```python
from build123d import *

# Parameters (mm, degrees)
SKETCH1_W           = 46.99
SKETCH1_H           = 12.7
SKETCH1_R           = 1.5875
SKETCH1_R_2         = 1.6129
BOSS_EXTRUDE1_DEPTH = 5.715
SKETCH2_R           = 2.921
CUT_EXTRUDE1_DEPTH  = 3.302
FILLET1_R           = 2.54
FILLET2_R           = 0.254


with BuildPart() as part:
    # Sketch1 → Boss-Extrude1 (new body)
    with BuildSketch(Plane(origin=(0, 0, 0), x_dir=(0, 0, -1), z_dir=(1, 0, 0))):
        Rectangle(SKETCH1_W, SKETCH1_H)
        with Locations((-19.05, 0)):
            Circle(SKETCH1_R, mode=Mode.SUBTRACT)
        with Locations(Location((19.05, 0, 0), (0, 0, 180))):
            Circle(SKETCH1_R, mode=Mode.SUBTRACT)
        with Locations((-4.028538113, -1.878538173)):
            Circle(SKETCH1_R_2, mode=Mode.SUBTRACT)
        with Locations((4.028538113, 1.878538173)):
            Circle(SKETCH1_R_2, mode=Mode.SUBTRACT)
    extrude(amount=BOSS_EXTRUDE1_DEPTH)

    # Sketch2 → Cut-Extrude1 (cut)
    with BuildSketch(Plane(origin=(5.715, 0, 0), x_dir=(0, 0, -1), z_dir=(1, 0, 0))):
        with Locations((-4.028538113, -1.878538173)):
            Circle(SKETCH2_R)
        with Locations((4.028538113, 1.878538173)):
            Circle(SKETCH2_R)
    extrude(amount=-CUT_EXTRUDE1_DEPTH, mode=Mode.SUBTRACT)

    # Fillet1
    fillet1_edges = [part.edges().sort_by_distance(p)[0] for p in [
        (2.8575, 6.35, 23.495),
        (2.8575, 6.35, -23.495),
        (2.8575, -6.35, -23.495),
        (2.8575, -6.35, 23.495),
    ]]
    fillet(fillet1_edges, radius=FILLET1_R)

    # Fillet2
    fillet2_edges = [part.edges().sort_by_distance(p)[0] for p in [
        (2.413, -1.878538173, 6.949538113),
        (2.413, 1.878538173, -1.107538113),
    ]]
    fillet(fillet2_edges, radius=FILLET2_R)


solid = part.part
```
Verification items for the finished model (mm, model axes). A direction names the side the tool comes from. Coordinates: 2 decimals unless noted, no trailing zeros. Write item = value, one per line.
Q1. Go/stop test with a flat-tipped pin: pin 1 Ø3.5 at (y, z) = (1.88, -4.03) entering from +X. Record where the tip stops, or that it passes through.
Answer:
pin_1 = 2.41
Q2. Cross-section at B-B (x = 4.6). Give the number of separate pieces and of enclosed holes in the cut face, plus the area to 3 significant figures.
Answer:
separate_pieces = 1
enclosed_holes = 4
area = 522 mm²
Q3. Mould release check, pull along Y, two halves, no side actions. Record for faces 3 (the face through (3, 0, 23.495)), 4 (the face through (4.21, 4.34, -5.6)), 5 (the face through (1.19, 2.97, -2.84)), 6 (the face through (2.898, -5.626, -22.731)): released by +Y, released by -Y, zero draft, split by the parting line, or undercut.
Answer:
face_3 = zero draft
face_4 = undercut
face_5 = undercut
face_6 = released by -Y
Q4. Access from +Z, -Z, +X, -X, +Y, -Y to the whole of each face (thin tool, end or side, straight path). Record for faces 1 (the face through (2.898, 5.586, 22.771)), 2 (the face through (2.413, -4, 4)).
Answer:
face_1 = +Z, +X, -X, +Y
face_2 = +X
Q5. Material ranges on L1, parallel to Z at x = 1.8, y = -1 (3 decimals); L2, parallel to Y at x = 3.15, z = -19.05; L3, parallel to Z at x = 5.5, y = -3.5 (3 decimals), recorded low to high. Write a range as from..to.
Answer:
L1 = -23.495..-20.283, -17.817..2.676, 5.381..17.817, 20.283..23.495
L2 = -6.35..-1.59, 1.59..6.35
L3 = -23.495..1.599, 6.458..23.495
